Check sheet for the modelled part. Datum: model origin and axes. Units: mm. A direction names the side the tool comes from. Coordinates: 2 decimals unless noted, no trailing zeros. Loops run counter-clockwise (first coordinate to the right, second up) from the corner with the lowest first, then second, coordinate; pieces in that order, holes last. Notation, with made-up numbers: M 54,1.25 L 81,1.25 A22 cw 81,8.25 Z; hole C 49.5,30.5 d11. An arc over 180 degrees is marked long. Answer in a Markdown table with one row per item. Add a question column.
Autodesk Inventor part; units mm, degrees
ref_plane "YZ Plane" through (0, 0, 0) normal (1, 0, 0) x (0, 1, 0)
ref_plane "XZ Plane" through (0, 0, 0) normal (0, 1, 0) x (-1, 0, 0)
ref_plane "XY Plane" through (0, 0, 0) normal (0, 0, 1) x (1, 0, 0)
sketch "Sketch20" plane through (0, 0, 0) normal (0, 1, 0) x (-1, 0, 0)
  line L0 (1.5185, -0.8925) -> (-3.5615, -0.8925)
  line L1 (-3.5615, -0.8925) -> (-3.5615, 11.8075)
  line L2 (-3.5615, 11.8075) -> (1.5185, 11.8075)
  line L3 (1.5185, 11.8075) -> (1.5185, -0.8925)
  line L4 (1.5185, 4.9634) -> (-3.5615, 4.9634)
  point P0 (0, 0)
  dimension "d56" = 5.08
  dimension "d57" = 12.7
extrude "Extrusion7" add sketch "Sketch20" along normal blind 2.54 contours L0 L1 L4 L3
extrude "Extrusion8" add sketch "Sketch20" along normal blind 6.35 contours L4 L1 L2 L3
sketch "Sketch21" plane through (0, 2.54, 0) normal (0, 1, 0) x (1, 0, 0)
  line L0 (3.5615, 0.8925) -> (-1.5185, 0.8925)
  line L1 (-1.5185, 0.8925) -> (-1.5185, -4.9634)
  point P0 (0, 0)
  point P1 (1.0215, -1.6475)
  dimension "d62" = 2.54
  dimension "d63" = 2.54
hole "Hole5" at (1.0215, 2.54, 1.6475) direction (0, -1, 0) diameter 2.4867 end through all
sketch "Sketch22" plane through (3.5615, 0, -0.8925) normal (1, 0, 0) x (0, 0, -1)
  line L0 (-12.7, 6.35) -> (-5.8558, 6.35)
  line L1 (-12.7, 0) -> (-12.7, 6.35)
  point P0 (-0.8925, 0)
  point P1 (-7.493, 3.175)
  dimension "d71" = 3.175
  dimension "d72" = 5.207
hole "Hole6" at (3.5615, 3.175, 6.6005) direction (-1, 0, 0) diameter 2.459 end through all
sketch "Sketch23" plane through (0, 2.54, 0) normal (0, 1, 0) x (1, 0, 0)
  line L0 (-1.5185, 0.8925) -> (-1.5185, -4.9634)
  line L1 (-1.5185, -4.9634) -> (-1.5185, -3.6934)
  line L2 (-1.5185, -3.6934) -> (3.5615, -3.6934)
  line L3 (3.5615, -4.9634) -> (3.5615, 0.8925)
  line L4 (3.5615, -3.6934) -> (3.5615, -4.9634)
  line L5 (3.5615, -11.8075) -> (3.5615, 0.8925)
  line L6 (3.5615, -4.9634) -> (-1.5185, -4.9634)
  line L7 (-1.5185, -4.9634) -> (3.5615, -4.9634)
  point P0 (0, 0)
  dimension "d80" = 1.27
extrude "Extrusion9" add sketch "Sketch23" along normal blind 3.81
sketch "Sketch25" plane through (3.5615, 0, -0.8925) normal (1, 0, 0) x (0, 0, -1)
  circle A0 centre (-7.493, 3.175) radius 1.2295
  line L0 (-7.493, 3.175) -> (-10.3886, 3.175)
  line L1 (-4.5858, 6.35) -> (-12.7, 6.35)
  line L2 (-12.7, 0) -> (0, 0)
  line L3 (-12.7, 6.35) -> (-10.3886, 6.35)
  line L4 (-10.3886, 6.35) -> (-10.3886, 0)
  line L5 (-10.3886, 0) -> (-12.7, 0)
  line L6 (-12.7, 0) -> (-12.7, 6.35)
  point P0 (-0.8925, 0)
  dimension "d83" = 2.8956
extrude "Extrusion10" cut sketch "Sketch25" against normal blind 25.4 contours L4 L2 L6 L1
properties part number "filament holders"
Q1. Mould release check, pull along Z, two halves, no side actions. Record for faces 3 (the face through (0.648, 1.252, 2.833)), 4 (the face through (3.562, 2, 4)), 5 (the face through (1, 3, 9.496)), 6 (the face through (0.99, 3.12, 7.83)): released by +Z, released by -Z, zero draft, split by the parting line, or undercut.
Q2. Go/stop test with flat-tipped pins: pin 1 (1.1 mm diameter, centred on x = 1.5, y = 5, fed in from -Z); pin 2 (2.5 mm diameter, centred on x = 0.5, z = 1, fed in from +Y). Record where each tip stops, or that it passes through.
Q3. Cross-section at A-A (x = 0). Count the separate pieces of the cut face and the enclosed holes in it, plus the area to 3 significant figures.
Q4. Access from +Z, -Z, +X, -X, +Y, -Y to the whole of each face (thin tool, end or side, straight path). Record for faces 1 (the face through (1, 0, 4)), 2 (the face through (0, 2.54, 0)).
Q5. Cross-section at B-B (y = 2.25). Record the cut outline in (x, z), plus the area to 3 significant figures.
Q6. Cross-section at C-C (z = 6). Record the cut outline in (x, y), plus the area to 3 significant figures.
Q7. Thickness scan on L1, parallel to Z at x = 2.65, y = 5.75; L2, parallel to Z at x = 1.1, y = 2.5; L3, parallel to Y at x = -0.8, z = 7.5. Record the ranges inside material, lowest first.
Answer key:
| question | item | result |
|---|---|---|
| 1 | face 3 | undercut |
| 1 | face 4 | zero draft |
| 1 | face 5 | released by +Z |
| 1 | face 6 | undercut |
| 2 | pin 1 | z = 3.69 |
| 2 | pin 2 | y = 2.54 |
| 3 | separate pieces | 2 |
| 3 | enclosed holes | 1 |
| 3 | area | 40.1 mm^2 |
| 4 | face 1 | +Z, -Z, +X, -X, -Y |
| 4 | face 2 | -Z, +X, -X, +Y |
| 5 | outline | M -1.52,-0.89 L 3.56,-0.89 L 3.56,5.79 L -1.52,5.79 Z; M -1.52,7.41 L 3.56,7.41 L 3.56,9.5 L -1.52,9.5 Z; hole C 1.02,1.65 d2.49 |
| 5 | area | 39.7 mm^2 |
| 6 | outline | M -1.52,0 L 3.56,0 L 3.56,2.1 L -1.52,2.1 Z; M -1.52,4.25 L 3.56,4.25 L 3.56,6.35 L -1.52,6.35 Z |
| 6 | area | 21.4 mm^2 |
| 7 | L1 | 3.69 to 9.5 |
| 7 | L2 | -0.89 to 0.41, 2.89 to 5.57, 7.63 to 9.5 |
| 7 | L3 | 0 to 2.34, 4.01 to 6.35 |
